Could you check a few things on this model? Use its own coordinates, in mm. A direction names the side the tool comes from. Coordinates: 2 decimals unless noted, no trailing zeros. Write each loop counter-clockwise with the first axis right and the second up, starting at its lowest first coordinate (ties: lowest second). Pieces come first, ordered by that corner, then holes.
Item 1: Which directions (+Z, -Z, +X, -X, +Y, -Y) give clear straight access to the entire face, cutting with the end or side of a thin tool? Please do faces 1 (the flat face through (0, 2, 0)), 2 (the flat face through (-36.276, 0.986, -35.895)), 3 (the cylindrical face through (-1.915, 1.31, -70.381)).
Item 2: I want a section at B-B on y = 1.5. Please give me the cut outline in (x, z), then the cut area to 3 significant figures.
Item 3: Thinking about a two-plate mould opening in Z: for faces 4 (the cylindrical face through (68.346, 1.31, 3.461)), 5 (the cylindrical face through (-87.454, 0.986, 4.636)), 6 (the flat face through (0, 0, 0)), which applies, +Z half, -Z half, draft (parallel to the pull), parting line (faces both ways), or undercut?
Item 4: I want a section at A-A on x = 0. Please give me the cut outline in (y, z), then the cut area to 3 significant figures.
Item 5: I want a section at C-C on z = 0. Please give me the cut outline in (x, y).
Item 6: If I drill on probe 1 along X at (y, z) = (1.65, 0); probe 2 along Z at (x, y) = (56, 0.3); probe 3 along X at (y, z) = (0.5, -41), over which ranges is the centre line in solid material (lowest first)?
Item 7: I want a section at D-D on x = -75. Please give me the cut outline in (y, z).
Item 8: For P1, Ø1, axis at x = -3.5, y = 0.5, coming from the -Z side; P2, Ø5, axis at x = 0.5, z = -76.5, coming from the +Y side, each with a flat end and sliding along its axis, tell me the tip position at first contact or that it passes through.
from build123d import *

# Parameters (mm, degrees)
AUFSATZ_LINEAR_AUSTRAGEN1_DEPTH = 2
SKIZZE2_R                       = 5
SKIZZE2_R_2                     = 10
SKIZZE2_R_3                     = 7.5
SCHNITT_LINEAR_AUSTRAGEN1_DEPTH = 1.4
VERRUNDUNG1_R                   = 2


with BuildPart() as part:
    # Skizze1 → Aufsatz-Linear austragen1 (new body)
    with BuildSketch(Plane(origin=(0, 0, 0), x_dir=(1, 0, 0), z_dir=(0, 1, 0))):
        with BuildLine():
            Line((-11.803204492, 66.025222633), (-67.124306483, 10.704120642))
            ThreePointArc((-67.124306483, 10.704120642), (-87.277686291, -5.085584176), (-61.862087415, -2))
            Line((-61.862087415, -2), (61.34027937, -2))
            ThreePointArc((61.34027937, -2), (87.754489642, -5.283082591), (66.755332476, 11.073094649))
            Line((66.755332476, 11.073094649), (11.803204492, 66.025222633))
            ThreePointArc((11.803204492, 66.025222633), (0, 89.827753204), (-11.803204492, 66.025222633))
        make_face()
        with BuildLine():
            Line((-8.974777367, 63.196795508), (-64.295879358, 7.875693517))
            ThreePointArc((-64.295879358, 7.875693517), (-62.722313709, 5.085584176), (-61.862087415, 2))
            Line((-61.862087415, 2), (61.34027937, 2))
            ThreePointArc((61.34027937, 2), (62.245510358, 5.283082591), (63.926905351, 8.244667524))
            Line((63.926905351, 8.244667524), (8.974777367, 63.196795508))
            ThreePointArc((8.974777367, 63.196795508), (0, 60.172246796), (-8.974777367, 63.196795508))
        make_face(mode=Mode.SUBTRACT)
    extrude(amount=AUFSATZ_LINEAR_AUSTRAGEN1_DEPTH)

    # Skizze2 → Schnitt-Linear austragen1 (cut)
    with BuildSketch(Plane(origin=(0, 2, 0), x_dir=(1, 0, 0), z_dir=(0, 1, 0))):
        with Locations(Location((0, 75, 0), (0, 0, 270))):
            Circle(SKIZZE2_R)
        with Locations(Location((-75, 0, 0), (0, 0, 270))):
            Circle(SKIZZE2_R_2)
        with Locations(Location((75, 0, 0), (0, 0, 270))):
            Circle(SKIZZE2_R_3)
    extrude(amount=-SCHNITT_LINEAR_AUSTRAGEN1_DEPTH, mode=Mode.SUBTRACT)

    # Verrundung1
    verrundung1_edges = [part.edges().sort_by_distance(p)[0] for p in [
        (-64.295879358, 1, -7.875693517),
        (-61.862087415, 1, -2),
        (61.34027937, 1, -2),
        (63.926905351, 1, -8.244667524),
        (8.974777367, 1, -63.196795508),
        (-8.974777367, 1, -63.196795508),
    ]]
    fillet(verrundung1_edges, radius=VERRUNDUNG1_R)


solid = part.part
Response values:
1. face 1: +Z, -Z, +X, -X, +Y
1. face 2: +Y, -Y
1. face 3: +Y
2. outline: (-67.12, -10.7) - (-11.8, -66.03) arc R14.83 ccw (long way) to (11.8, -66.03) - (66.76, -11.07) arc R13.81 ccw (long way) to (61.34, 2) - (-61.86, 2) arc R13.29 ccw (long way) to start; hole circle Ø20 at (-75, 0); hole (-63.47, -6.61) arc R2 ccw to (-63.15, -9.02) - (-10.14, -62.03) arc R2 ccw to (-7.69, -62.32) arc R14.83 cw to (7.69, -62.32) arc R2 ccw to (10.14, -62.03) - (62.77, -9.4) arc R2 ccw to (63.09, -6.97) arc R13.81 cw to (61.64, -3.49) arc R2 ccw to (59.71, -2) - (-60.24, -2) arc R2 ccw to (-62.17, -3.48) arc R13.29 cw to start; hole circle Ø10 at (0, -75); hole circle Ø15 at (75, 0)
2. area: 2,390 mm2
3. face 4: undercut
3. face 5: parting line
3. face 6: draft
4. outline: (0, -89.83) - (2, -89.83) - (2, -80) - (0.6, -80) - (0.6, -70) - (2, -70) - (2, -60.17) - (0, -60.17) - close; (0, -2) - (2, -2) - (2, 2) - (0, 2) - close
4. area: 53.3 mm2
5. outline: (-88.29, 0) - (88.81, 0) - (88.81, 2) - (82.5, 2) - (82.5, 0.6) - (67.5, 0.6) - (67.5, 2) - (-65, 2) - (-65, 0.6) - (-85, 0.6) - (-85, 2) - (-88.29, 2) - close
6. probe 1: x = -88.29 to -85, -65 to 67.5, 82.5 to 88.81
6. probe 2: z = -21.83 to -16.17, -2 to 2
6. probe 3: x = -36.83 to -31.17, 31.17 to 36.83
7. outline: (0, -13.29) - (2, -13.29) - (2, -10) - (0.6, -10) - (0.6, 10) - (2, 10) - (2, 13.29) - (0, 13.29) - close
8. P1: stops at z = -89.52
8. P2: stops at y = 0.6
